The figure shows three views and two pictorial views of one solid part (mm, origin at its lowest corner). Answer the questions. Round coordinates to 2 decimals unless told otherwise and drop trailing zeros. Write each loop counter-clockwise with the first axis right and the second up, starting at its lowest first coordinate (ties: lowest second). Pieces come first, ordered by that corner, then holes. Notation, with made-up numbers: M 2.25,-28.75 L 27.25,-28.75 A32 ccw 27.25,1.25 Z; hole C 87.25,-8 d2. An arc over 180 degrees is marked long. Answer in a Markdown table with one row per item.
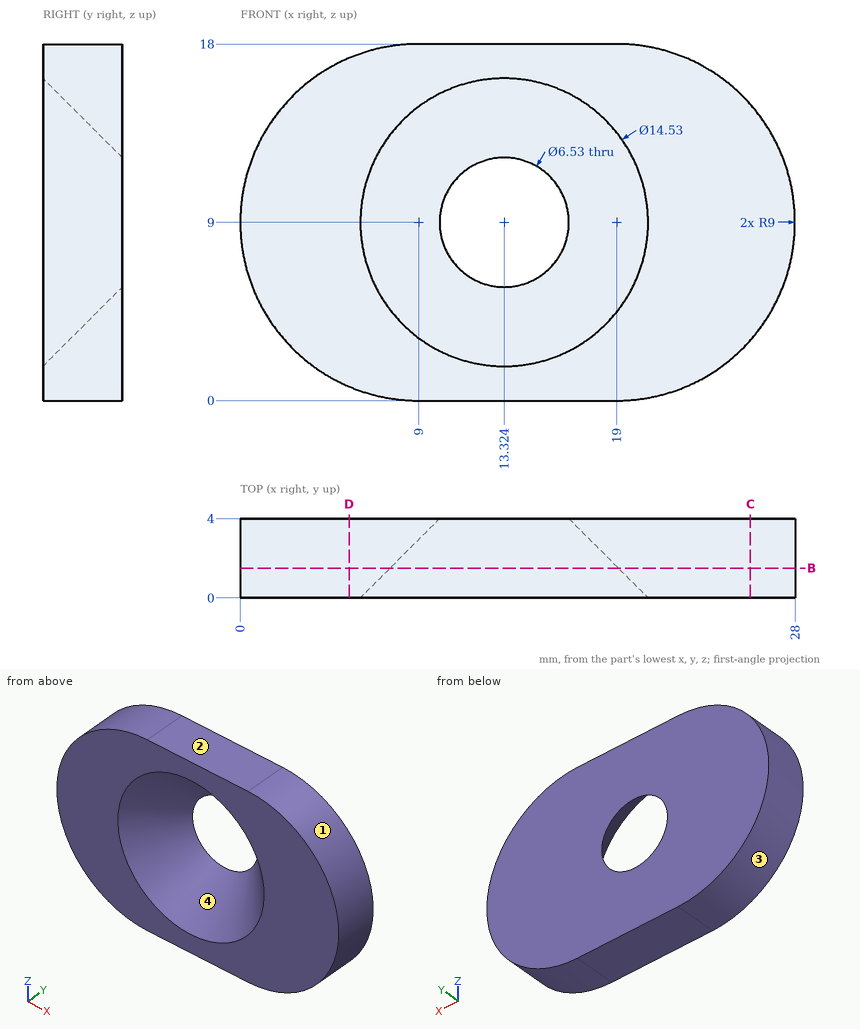
1. Given pin 1 (6 mm diameter, centred on x = 13.32, z = 9, fed in from -Y); pin 2 (2 mm diameter, centred on y = 3, z = 2.5, fed in from +X) (1 decimal), each flat-ended and moving along its own axis, determine where each tip first touches the part or whether it passes through.
Calculated:
| item | result |
|---|---|
| pin 1 | passes through |
| pin 2 | stops at x = 26.1 |
2. Consider line 1 along X through (y, z) = (2.6, 11) (1 decimal); line 2 along X through (y, z) = (2.4, 8.25); line 3 along Z through (x, y) = (14, 0.8). Determine where each line is inside the solid, lowest interval first. Write a range as from..to.
Calculated:
| item | result |
|---|---|
| line 1 | x = 0.2..9.1, 17.5..27.8 |
| line 2 | x = 0.03..8.52, 18.13..27.97 |
| line 3 | z = 0..2.57, 15.43..18 |
3. Determine the mould class of the marked faces 1, 2, 3 and 4 for opening direction X: released by +X, released by -X, zero draft, split by the parting line, or undercut.
Calculated:
| item | result |
|---|---|
| face 1 | released by +X |
| face 2 | zero draft |
| face 3 | released by -X |
| face 4 | undercut |
4. The part is cut by section D-D (x = 5.5). Determine the outline of the cut face in (y, z).
Calculated:
| item | result |
|---|---|
| outline | M 0,0.71 L 4,0.71 L 4,17.29 L 0,17.29 Z |
5. The part is cut by section B-B (y = 1.5). Determine the outline of the cut face in (x, z) (1 decimal).
Calculated:
| item | result |
|---|---|
| outline | M 9,0 L 19,0 A9 ccw 19,18 L 9,18 A9 ccw Z; hole C 13.3,9 d11.5 |
6. The part is cut by section C-C (x = 25.75). Determine the outline of the cut face in (y, z), plus the area to 3 significant figures.
Calculated:
| item | result |
|---|---|
| outline | M 0,3.05 L 4,3.05 L 4,14.95 L 0,14.95 Z |
| area | 47.6 mm² |
